Autodesk Inventor part; units mm, degrees
ref_plane "YZ Plane" through (0, 0, 0) normal (1, 0, 0) x (0, 1, 0)
ref_plane "XZ Plane" through (0, 0, 0) normal (0, 1, 0) x (-1, 0, 0)
ref_plane "XY Plane" through (0, 0, 0) normal (0, 0, 1) x (1, 0, 0)
sketch "Sketch1" plane through (0, 0, 0) normal (0, 0, 1) x (1, 0, 0)
  circle A0 centre (57.407, 53.064) radius 2.5
  circle A1 centre (57.407, 53.064) radius 10
  circle A2 centre (13.407, 27.6606) radius 2.5
  circle A3 centre (13.407, 27.6606) radius 10
  circle A4 centre (57.407, 2.2572) radius 2.5
  circle A5 centre (57.407, 2.2572) radius 10
  line L0 (25.407, -164.9104) -> (25.407, 85.0896) construction
  arc A6 (64.907, 53.064) -> (53.9811, 59.7359) centre (57.407, 53.064) ccw
  arc A7 (58.5116, -5.161) -> (64.907, 2.2572) centre (57.407, 2.2572) ccw
  line L1 (10.407, 27.6606) -> (16.407, 27.6606) construction
  line L2 (10.407, 25.0106) -> (16.407, 25.0106)
  line L3 (16.407, 30.3106) -> (10.407, 30.3106)
  arc A8 (10.407, 30.3106) -> (10.407, 25.0106) centre (10.407, 27.6606) ccw
  arc A9 (16.407, 25.0106) -> (16.407, 30.3106) centre (16.407, 27.6606) ccw
  circle A10 centre (10.407, 2.8412) radius 10
  arc A11 (-3.8238, 7.5832) -> (12.6162, -11.9952) centre (10.407, 2.8412) ccw
  line L4 (12.6162, -11.9952) -> (58.5116, -5.161)
  line L5 (53.9811, 59.7359) -> (8.8392, 36.5564)
  line L6 (64.907, 2.2572) -> (64.907, 53.064)
  line L7 (3.9198, 30.8219) -> (-3.8238, 7.5832)
  line L8 (-3.8238, 7.5832) -> (-11.5466, -15.5932) construction
  line L9 (12.6162, -11.9952) -> (-11.5466, -15.5932) construction
  line L10 (-11.5466, -15.5932) -> (31.917, 20.9033) construction
  line L11 (-8.093, 51.8526) -> (-8.093, -0.1388) construction
  circle A12 centre (-8.093, 38.8412) radius 3.5 construction
  circle A13 centre (-8.093, 2.8412) radius 3.5 construction
  line L12 (-20.593, 53.8412) -> (-4.593, 53.8412) construction
  line L13 (-4.593, 53.8412) -> (-4.593, -12.1588) construction
  line L14 (-4.593, -12.1588) -> (-20.593, -12.1588) construction
  line L15 (-20.593, -12.1588) -> (-20.593, 53.8412) construction
  line L16 (-20.593, 20.8412) -> (-4.593, 20.8412) construction
  line L17 (-2.413, 11.817) -> (-10.2687, 5.5829)
  line L18 (-10.2687, 0.0996) -> (1.0826, -8.9085)
  arc A14 (-4.593, -1.7035) -> (-4.0348, -1.2128) centre (-8.093, 2.8412) ccw
  arc A15 (-10.2687, 5.5829) -> (-10.2687, 0.0996) centre (-8.093, 2.8412) ccw
  line L19 (1.8905, 24.7319) -> (-10.4816, 36.2829)
  line L20 (-7.3703, 42.2658) -> (11.9978, 38.1783)
  arc A16 (-7.3703, 42.2658) -> (-10.4816, 36.2829) centre (-8.093, 38.8412) ccw
  point P0 (18.407, 14.782)
  point P1 (23.5514, 8.6555)
  dimension "d52" = 15
  dimension "d53" = 15
  dimension "d54" = 3
  dimension "d55" = 5.3
  dimension "d56" = 20
  dimension "d57" = 30
  dimension "d58" = 4
  dimension "d59" = 8
  dimension "d93" = 7
  dimension "d94" = 7
  dimension "d95" = 36
  dimension "d96" = 16
  dimension "d97" = 66
  dimension "d99" = 3.5
extrude "Extrusion1" add sketch "Sketch1" along normal blind 4 contours A0 | L5 A6 L6 A1 | A1 L6 A5 L4 A11 L7 A3 L5 | L5 A3 L7 L19 A16 L20 | L6 A7 L4 A5 | A3 | L18 A15 L17 L7 A11 | A4 picked at (52.4239, 56.8921) picked at (55.6672, -3.7922)
sketch "Sketch2" plane through (0, 0, 4) normal (0, 0, 1) x (1, 0, 0)
  circle A0 centre (13.407, 27.6606) radius 2.5
  circle A1 centre (57.407, 2.2572) radius 2.5
  circle A2 centre (57.407, 53.064) radius 2.5
  line L0 (10.407, 27.6606) -> (16.407, 27.6606) construction
  line L1 (10.407, 24.9106) -> (16.407, 24.9106)
  line L2 (16.407, 30.4106) -> (10.407, 30.4106)
  arc A3 (10.407, 30.4106) -> (10.407, 24.9106) centre (10.407, 27.6606) ccw
  arc A4 (16.407, 24.9106) -> (16.407, 30.4106) centre (16.407, 27.6606) ccw
  point P0 (0, 0)
  dimension "d25" = 3
  dimension "d26" = 5.5
hole "Hole2" at (57.407, 53.064, 4) at (57.407, 2.2572, 4) direction (0, 0, -1) diameter 5.5 end through all
hole "Hole4" at (18.407, 14.782, 0) at (23.5514, 8.6555, 0) direction (0, 0, 1) diameter 3 end through all
sketch "Sketch6" plane through (0, 0, 0) normal (0, 0, -1) x (-1, 0, 0)
  circle A0 centre (-49.2903, 15.4803) radius 1.7
  circle A1 centre (-30.2236, 38.1868) radius 1.7
  point P0 (0, 0)
hole "Hole6" at (49.2903, 15.4803, 0) at (30.2236, 38.1868, 0) direction (0, 0, 1) diameter 3.4 end through all countersink diameter 6.6 countersink angle 90
sketch "Sketch7" plane through (0, 0, 4) normal (0, 0, 1) x (1, 0, 0)
  point P0 (0, 0)
  point P1 (49.6217, 42.3118)
  point P2 (59.6217, 42.3118)
hole "Hole7" at (59.6217, 42.3118, 4) at (49.6217, 42.3118, 4) direction (0, 0, -1) diameter 3.4 end through all countersink diameter 6.6 countersink angle 90
hole "Hole8" at (-8.093, 2.8412, 0) at (-8.093, 38.8412, 0) direction (0, 0, 1) diameter 3.4 end through all
fillet "Fillet2" radius 5 3 edges at (-2.413, 11.817, 2) (1.8905, 24.7319, 2) (11.9978, 38.1783, 2)
properties part number "plate_3"
Geometry: final body of the model. Coordinates: model frame, mm. A direction names the side the tool comes from. Give positions to 0.01 mm unless a question says otherwise; leave off trailing zeros. Write each loop counter-clockwise with the first axis right and the second up, starting at its lowest first coordinate (ties: lowest second). Pieces come first, ordered by that corner, then holes. Notation, with made-up numbers: M -8,-16.75 L 2,-16.75 A21 cw 2,20.25 Z; hole C 17.5,-1.75 d7. An arc over 180 degrees is marked long. Answer in a Markdown table with one row per item. Add a question column.
(1) Section A-A on x = 15.5. Return loops of the section in (y, z), and give its area (3 significant figures).
(2) Mould query, pull axis Y, two halves, no side actions, for faces 1 (the flat face through (1.32, 40.43, 1.97)), 2 (the cylindrical face through (29.075, 36.934, 2.817)), 3 (the flat face through (35, 25, 0)), 4 (the flat face through (-4.673, -4.341, 1.972)). Classes: +Y half, -Y half, draft (parallel to the pull), parting line (faces both ways), or undercut.
(3) First-contact query: pin 1 (1.5 mm diameter, centred on x = 29.5, z = 2.5, fed in from +Y); pin 2 (4 mm diameter, centred on x = -8.09, y = 2.84, fed in from -Z); pin 3 (1.2 mm diameter, centred on x = 12, z = 2.5, fed in from -Y); pin 4 (1 mm diameter, centred on y = 24, z = 3, fed in from -X). Flat tips, straight axial feed; report the tip coordinate or a pass-through.
(4) Ray query, line 1 (Y direction, x = 10.5, z = 0.95); line 2 (X direction, y = 9.5, z = 1.1); line 3 (X direction, y = 13, z = 0.4). Return the intervals inside material, ascending.
(5) Reachability of faces 5 (the flat face through (-5.4, 31.54, 1.97)), 6 (the flat face through (13, 25.011, 2)), 7 (the cylindrical face through (63.14, -2.58, 1.97)) from +Z, -Z, +X, -X, +Y, -Y: full face, straight path, thin tool, end or side. Return the list, or none.
(6) Section C-C on x = 39.5. Return loops of the section in (y, z), and give its area (3 significant figures).
(7) Section B-B on z = 0.85. State how many separate pieces and enclosed holes the cut face has, and give its area (3 significant figures).
Result set:
| question | item | result |
|---|---|---|
| 1 | outline | M -11.57,0 L -5.76,0 L -5.76,4 L -11.57,4 Z; M 11.45,0 L 25.01,0 L 25.01,4 L 11.45,4 Z; M 30.31,0 L 39.98,0 L 39.98,4 L 30.31,4 Z |
| 1 | area | 116 mm^2 |
| 2 | face 1 | +Y half |
| 2 | face 2 | undercut |
| 2 | face 3 | draft |
| 2 | face 4 | -Y half |
| 3 | pin 1 | stops at y = 47.55 |
| 3 | pin 2 | stops at z = 0 |
| 3 | pin 3 | stops at y = -12.13 |
| 3 | pin 4 | stops at x = 0.98 |
| 4 | line 1 | y = -12.16 to -7.16, 12.84 to 25.01, 30.31 to 38.5 |
| 4 | line 2 | x = -5.33 to 2.95, 17.87 to 22.31, 24.79 to 64.91 |
| 4 | line 3 | x = -2.03 to 47.79, 50.79 to 64.91 |
| 5 | face 5 | +Z, -Z, -X |
| 5 | face 6 | +Z, -Z |
| 5 | face 7 | +Z, -Z, +X, -Y |
| 6 | outline | M -7.99,0 L 52.3,0 L 52.3,4 L -7.99,4 Z |
| 6 | area | 241 mm^2 |
| 7 | separate pieces | 1 |
| 7 | enclosed holes | 12 |
| 7 | area | 3,490 mm^2 |
